from build123d import *

# Parameters (mm, degrees)
BASPROSKE_W         = 10
BASPROSKE_H         = 25.875
TOOTHCUT_DEPTH      = 38.934565372
TEETHCUTS_COUNT     = 21
TEETHCUTS_ANGLE     = 342.857142857
BORSKE_R            = 11
BORE_DEPTH          = 50.0000508
SKETCH2_R           = 11
BOSS_EXTRUDE2_DEPTH = 3


with BuildPart() as part:
    # BasProSke → Base-Revolve (revolve)
    with BuildSketch(Plane(origin=(0, 0, 0), x_dir=(1, 0, 0), z_dir=(0, 1, 0)), mode=Mode.PRIVATE) as base_revolve_sk:
        with Locations((5, 12.9375)):
            Rectangle(BASPROSKE_W, BASPROSKE_H)
    revolve(base_revolve_sk.sketch.rotate(Axis((-10, 0, 0), (1, 0, 0)), 180), axis=Axis((-10, 0, 0), (1, 0, 0)))

    # TooCutSke → ToothCut (cut, through all)
    with BuildSketch(Plane(origin=(0, 0, 0), x_dir=(0, 0, -1), z_dir=(1, 0, 0))):
        with BuildLine():
            ThreePointArc((1.101400125, 20.782335047), (0, 20.8115), (-1.101400125, 20.782335047))
            ThreePointArc((-1.101400125, 20.782335047), (-1.83071474, 23.395008735), (-3.272169586, 25.692871119))
            ThreePointArc((-3.272169586, 25.692871119), (0, 25.9004), (3.272169586, 25.692871119))
            ThreePointArc((3.272169586, 25.692871119), (1.83071474, 23.395008735), (1.101400125, 20.782335047))
        make_face()
    toothcut = extrude(amount=TOOTHCUT_DEPTH, mode=Mode.SUBTRACT)

    # TeethCuts: ToothCut ×21 about axis
    teethcuts_axis = Axis((-10, 0, 0), (1, 0, 0))
    for i in range(1, TEETHCUTS_COUNT):
        add(toothcut.rotate(teethcuts_axis, i * TEETHCUTS_ANGLE / (TEETHCUTS_COUNT - 1)), mode=Mode.SUBTRACT)

    # BorSke → Bore (cut, symmetric)
    with BuildSketch(Plane(origin=(0, 0, 0), x_dir=(0, 0, -1), z_dir=(1, 0, 0))):
        with Locations(Location((0, 0, 0), (0, 0, 180))):
            Circle(BORSKE_R)
    extrude(amount=BORE_DEPTH, both=True, mode=Mode.SUBTRACT)

    # Sketch2 → Boss-Extrude2 (add)
    with BuildSketch(Plane(origin=(10, 0, 0), x_dir=(0, 0, -1), z_dir=(1, 0, 0))):
        Circle(SKETCH2_R)
    extrude(amount=-BOSS_EXTRUDE2_DEPTH)


solid = part.part
CAD build for the part. Positions are in the model's coordinates, mm. A direction names the side the tool comes from. Coordinates: 2 decimals unless noted, no trailing zeros. Order: outer loops, then holes, each group sorted by start corner. A loop starts at its lowest first (then second) coordinate and runs counter-clockwise, first axis right, second up.
Item 1: Band-saw the part on A-A on z = 0. List the corners of the cut face in (x, y) (1 decimal).
Check sheet entries:
outline: (0, -25.9) - (10, -25.9) - (10, 20.8) - (0, 20.8) - (0, 11) - (7, 11) - (7, -11) - (0, -11) - close
Item 2: Drill centre lines: L1, parallel to Y at x = 3, z = 0 (1 decimal); L2, parallel to Z at x = 8, y = 21; L3, parallel to Z at x = 2, y = -4.5. Where is each one in solid material? Low to high.
Check sheet entries:
L1: y = -25.9 to -11, 11 to 20.8
L2: z = -11.76 to -8.01, -5.18 to -1.13, 1.13 to 5.18, 8.01 to 11.76
L3: z = -20.32 to -10.04, 10.04 to 20.32
Item 3: Two-plate mould, pull along Y, no slides. Class faces 1 (the face through (5.07, 25.585, -3.865)), 2 (the face through (4.93, 15.971, -17.125)), 3 (the face through (5.07, -24.723, 7.635)): +Y half, -Y half, draft (parallel to the pull), parting line (faces both ways), or undercut.
Check sheet entries:
face 1: +Y half
face 2: undercut
face 3: -Y half
Item 4: 3-axis set-ups, long thin cutter, end or side, ignore diameter. For faces 4 (the face through (4.93, -13.3, -19.36)), 5 (the face through (4.93, -6.96, 22.36)), 6 (the face through (4.93, -10.392, 18.031)): which of +Z, -Z, +X, -X, +Y, -Y reach the whole face in a straight line?
Check sheet entries:
face 4: -Z, +X, -X
face 5: +Z, +X, -X
face 6: +X, -X
Item 5: Pin check, flat tips, straight feed: pin 1 Ø6 at (x, z) = (2.5, -7.5) entering from +Y; pin 2 Ø3 at (x, z) = (8, -18.5) entering from -Y; pin 3 Ø5 at (x, z) = (4.5, 3) entering from +Y. Stop position of each tip, or through.
Check sheet entries:
pin 1: stops at y = 25.39
pin 2: stops at y = -16.6
pin 3: stops at y = 25.67
